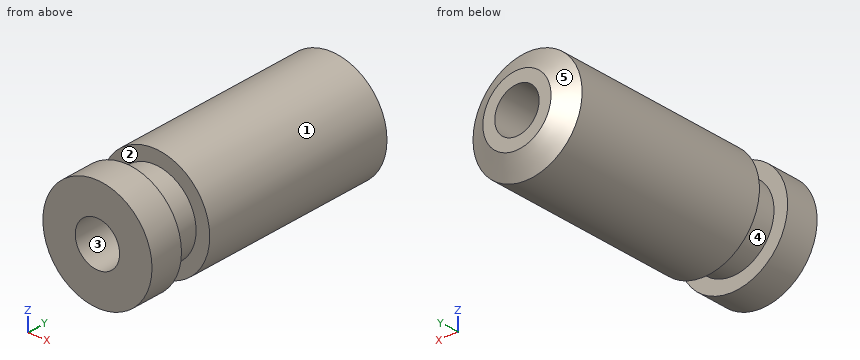
```python
from build123d import *

# Parameters (mm, degrees)
SKETCH3_R          = 3.25
CUT_EXTRUDE1_DEPTH = 41


with BuildPart() as part:
    # Sketch2 → Revolve1 (revolve)
    with BuildSketch(Plane.XY):
        Polygon((0, 0), (8, 0), (8, 4.8), (6, 4.8), (6, 9.4), (8, 9.4), (8, 38.267949192), (5, 40), (0, 40), align=None)
    revolve(axis=Axis((0, 40, 0), (0, -1, 0)))

    # Sketch3 → Cut-Extrude1 (cut, through all)
    with BuildSketch(Plane.XZ):
        Circle(SKETCH3_R)
    extrude(amount=-CUT_EXTRUDE1_DEPTH, mode=Mode.SUBTRACT)


solid = part.part
```
Could you check a few things on this model? Use its own coordinates, in mm. Face numbers are marked on the shaded views. A direction names the side the tool comes from. Round coordinates to 2 decimals unless told otherwise and drop trailing zeros. Loops run counter-clockwise (first coordinate to the right, second up) from the corner with the lowest first, then second, coordinate; pieces in that order, holes last. Notation, with made-up numbers: (89.25, -35.75) -> (115.25, -35.75) arc R23 cw to (115.25, 1.25) -> close; hole circle Ø11 at (85.25, -10.75). An arc over 180 degrees is marked (long way). One line per question, with ' | ' between items.
(1) If I drill on probe 1 along Z at (x, y) = (0, 10); probe 2 along X at (y, z) = (20.5, -6.25); probe 3 along Y at (x, z) = (-5.75, -5.5), over which ranges is the centre line in solid material (lowest first)?
Model answer:
probe 1: z = -8 to -3.25, 3.25 to 8 | probe 2: x = -4.99 to 4.99 | probe 3: y = 0 to 4.8, 9.4 to 38.29
(2) Thinking about a two-plate mould opening in Z: for the marked faces 1, 2 and 3, which applies, released by +Z, released by -Z, zero draft, split by the parting line, or undercut?
Model answer:
face 1: split by the parting line | face 2: zero draft | face 3: undercut
(3) If we section it at A-A on x = 0: List the corners of the cut face in (y, z) for me, and give its area (3 significant figures).
Model answer:
outline: (0, -8) -> (4.8, -8) -> (4.8, -6) -> (9.4, -6) -> (9.4, -8) -> (38.27, -8) -> (40, -5) -> (40, -3.25) -> (0, -3.25) -> close; (0, 3.25) -> (40, 3.25) -> (40, 5) -> (38.27, 8) -> (9.4, 8) -> (9.4, 6) -> (4.8, 6) -> (4.8, 8) -> (0, 8) -> close | area: 356 mm^2
(4) If we section it at C-C on y = 21: List the corners of the cut face in (x, z) for me.
Model answer:
outline: circle Ø16 at (0, 0); hole circle Ø6.5 at (0, 0)
(5) If we section it at B-B on z = 0: List the corners of the cut face in (x, y) for me, and give its area (3 significant figures).
Model answer:
outline: (-8, 0) -> (-3.25, 0) -> (-3.25, 40) -> (-5, 40) -> (-8, 38.27) -> (-8, 9.4) -> (-6, 9.4) -> (-6, 4.8) -> (-8, 4.8) -> close; (3.25, 0) -> (8, 0) -> (8, 4.8) -> (6, 4.8) -> (6, 9.4) -> (8, 9.4) -> (8, 38.27) -> (5, 40) -> (3.25, 40) -> close | area: 356 mm^2
(6) For pin 1 Ø3 at (y, z) = (24, 2) entering from +X; pin 2 Ø8 at (x, z) = (2, -6) entering from +Y; pin 3 Ø2 at (y, z) = (30, -6) entering from +X (3 decimals); pin 4 Ø1.5 at (x, y) = (5, 28.5) entering from +Z, each with a flat end and sliding along its axis, tell me the tip position at first contact or that it passes through.
Model answer:
pin 1: stops at x = 7.98 | pin 2: stops at y = 40 | pin 3: stops at x = 6.245 | pin 4: stops at z = 6.78
(7) For the marked faces 4 and 5, which set-ups out of +Z, -Z, +X, -X, +Y, -Y let a thin tool reach every point of the face, with its end or its side?
Model answer:
face 4: none | face 5: +Y
(8) If we section it at D-D on y = 7.5: List the corners of the cut face in (x, z) for me, and give its area (3 significant figures).
Model answer:
outline: circle Ø12 at (0, 0); hole circle Ø6.5 at (0, 0) | area: 79.9 mm^2
